Geometry check sheet. Reference: the model listing, model coordinates, mm. A direction names the side the tool comes from. Round coordinates to 2 decimals unless told otherwise and drop trailing zeros. Loops run counter-clockwise (first coordinate to the right, second up) from the corner with the lowest first, then second, coordinate; pieces in that order, holes last. Notation, with made-up numbers: M -31,84.25 L -17,84.25 A16 cw -17,107.25 Z; hole C 6.25,13.25 d8. An arc over 180 degrees is marked long. Answer in a Markdown table with one row per item. Add a question column.
```python
from build123d import *

# Parameters (mm, degrees)
SKETCH_1_R                = 31.85
EXTRUDE_1_DEPTH           = 18
SKETCH_2_R                = 25
SKETCH_2_R_2              = 9
CUT_EXTRUDE_1_DEPTH       = 6.2
CUT_EXTRUDE_START         = -6.2
SKETCH_3_R                = 25
SKETCH_3_R_2              = 9
CUT_EXTRUDE_5_DEPTH       = 6.2
EXTRUDE_START             = 9
SKETCH_4_R                = 9
EXTRUDE_2_DEPTH           = 9
SKETCH_5_R                = 3
CUT_EXTRUDE_6_DEPTH       = 53.515188279
SKETCH_6_R                = 6
CUT_EXTRUDE_7_DEPTH       = 48.538247759
CUT_EXTRUDE_10_REACH      = 60.414
CUT_EXTRUDE_10_END_RADIUS = 3
SKETCH_10_R               = 2
CUT_EXTRUDE_11_REACH      = 60.414
CUT_EXTRUDE_11_END_RADIUS = 3
SKETCH_7_R                = 2


with BuildPart() as part:
    # 草图1 → 凸台-拉伸1 (new body)
    with BuildSketch(Plane.XY):
        Circle(SKETCH_1_R)
    extrude(amount=EXTRUDE_1_DEPTH)

    # 草图2 → 切除-拉伸1 (cut)
    with BuildSketch(Plane.XY.offset(18)):
        Circle(SKETCH_2_R)
        Circle(SKETCH_2_R_2, mode=Mode.SUBTRACT)
    extrude(amount=-CUT_EXTRUDE_1_DEPTH, mode=Mode.SUBTRACT)

    # 草图3 → 切除-拉伸5 (cut)
    with BuildSketch(Plane(origin=(0, 0, 0), x_dir=(-1, 0, 0), z_dir=(0, 0, -1)).offset(CUT_EXTRUDE_START)):
        with Locations(Location((0, 0, 0), (0, 0, 180))):
            Circle(SKETCH_3_R)
        with Locations(Location((0, 0, 0), (0, 0, 180))):
            Circle(SKETCH_3_R_2, mode=Mode.SUBTRACT)
    extrude(amount=CUT_EXTRUDE_5_DEPTH, mode=Mode.SUBTRACT)

    # 草图4 → 凸台-拉伸2 (add)
    with BuildSketch(Plane.XY.offset(18).offset(EXTRUDE_START)):
        Circle(SKETCH_4_R)
    extrude(amount=-EXTRUDE_2_DEPTH)

    # 草图5 → 切除-拉伸6 (cut, through all)
    with BuildSketch(Plane.XY.offset(27)):
        Circle(SKETCH_5_R)
    extrude(amount=-CUT_EXTRUDE_6_DEPTH, mode=Mode.SUBTRACT)

    # 草图6 → 切除-拉伸7 (cut, through all)
    with BuildSketch(Plane.XY.offset(11.8)):
        with Locations((-17, 0)):
            Circle(SKETCH_6_R)
        with Locations((-8.5, 14.722431864)):
            Circle(SKETCH_6_R)
        with Locations((8.5, 14.722431864)):
            Circle(SKETCH_6_R)
        with Locations((17, 0)):
            Circle(SKETCH_6_R)
        with Locations((8.5, -14.722431864)):
            Circle(SKETCH_6_R)
        with Locations((-8.5, -14.722431864)):
            Circle(SKETCH_6_R)
    extrude(amount=-CUT_EXTRUDE_7_DEPTH, mode=Mode.SUBTRACT)

    # 切除-拉伸10: up to this cylinder (the profile starts outside it)
    cut_extrude_10_end = Plane(origin=(0, 0, 19.4), z_dir=(0, 0, 1)) * Cylinder(CUT_EXTRUDE_10_END_RADIUS, 127.828, mode=Mode.PRIVATE)
    # 草图10 → 切除-拉伸10 (cut, up to the surface)
    with BuildSketch(Plane(origin=(0, 9, 0), x_dir=(1, 0, 0), z_dir=(0, 1, 0)), mode=Mode.PRIVATE) as cut_extrude_10_sk1:
        with Locations(Location((0, -19.4, 0), (0, 0, 270))):
            Circle(SKETCH_10_R)
    cut_extrude_10_tool1 = extrude(cut_extrude_10_sk1.sketch, amount=-CUT_EXTRUDE_10_REACH, mode=Mode.PRIVATE) - cut_extrude_10_end
    add(cut_extrude_10_tool1.solids().sort_by_distance((0, 9, 19.4))[0], mode=Mode.SUBTRACT)

    # 切除-拉伸11: up to this cylinder (the profile starts outside it)
    cut_extrude_11_end = Plane(origin=(0, 0, 19.4), z_dir=(0, 0, 1)) * Cylinder(CUT_EXTRUDE_11_END_RADIUS, 127.828, mode=Mode.PRIVATE)
    # 草图7 → 切除-拉伸11 (cut, up to the surface)
    with BuildSketch(Plane(origin=(9, 0, 0), x_dir=(0, 0, -1), z_dir=(1, 0, 0)), mode=Mode.PRIVATE) as cut_extrude_11_sk1:
        with Locations((-19.4, 0)):
            Circle(SKETCH_7_R)
    cut_extrude_11_tool1 = extrude(cut_extrude_11_sk1.sketch, amount=-CUT_EXTRUDE_11_REACH, mode=Mode.PRIVATE) - cut_extrude_11_end
    add(cut_extrude_11_tool1.solids().sort_by_distance((9, 0, 19.4))[0], mode=Mode.SUBTRACT)


solid = part.part
```
1) Cross-section at A-A, the plane y = -15.5. Record the boundary of the cut face in (x, z).
2) Cross-section at D-D, the plane x = -20. Record the boundary of the cut face in (y, z), plus the area to 3 significant figures.
3) Cross-section at C-C, the plane y = 4.5. Count the separate pieces of the cut face and the enclosed holes in it, plus the area to 3 significant figures.
4) Go/stop test with flat-tipped pins: pin 1 (8 mm diameter, centred on x = -1.5, z = 4, fed in from -Y); pin 2 (2 mm diameter, centred on x = -15, z = 7.5, fed in from -Y); pin 3 (1 mm diameter, centred on y = -5, z = 20, fed in from +X). Record where each tip stops, or that it passes through.
5) Draft check along Y on faces 4 (the cylindrical face through (7.199, 8.865, 9.039)), 5 (the cylindrical face through (30.38, 9.57, 8.87)), 6 (the flat face through (0, -4, 0)). Enter one of: +Y half, -Y half, draft (parallel to the pull), parting line (faces both ways), or undercut.
6) Set-up check for faces 1 (the cylindrical face through (-0.766, 5.666, 21.247)), 2 (the cylindrical face through (23.846, 7.509, 14.943)), 3 (the flat face through (10.8, -0.4, 6.2)): record each of +Z, -Z, +X, -X, +Y, -Y from which the full face is reachable in a straight line by a thin tool's end or side.
7) Thickness scan on L1, parallel to Y at x = 0, z = 2.25; L2, parallel to Y at x = 8.5, z = 7.65; L3, parallel to Y at x = -12, z = 9.25. Record the ranges inside material, lowest first. Write a range as [from, to].
8) Cross-section at B-B, the plane x = -13. Record the boundary of the cut face in (y, z).
Worked answers:
| question | item | result |
|---|---|---|
| 1 | outline | M -27.82,0 L -19.62,0 L -19.62,6.2 L -14.45,6.2 L -14.45,11.8 L -19.62,11.8 L -19.62,18 L -27.82,18 Z; M -2.55,6.2 L 2.55,6.2 L 2.55,11.8 L -2.55,11.8 Z; M 14.45,6.2 L 19.62,6.2 L 19.62,0 L 27.82,0 L 27.82,18 L 19.62,18 L 19.62,11.8 L 14.45,11.8 Z |
| 2 | outline | M -24.79,0 L -15,0 L -15,6.2 L -5.2,6.2 L -5.2,11.8 L -15,11.8 L -15,18 L -24.79,18 Z; M 5.2,6.2 L 15,6.2 L 15,0 L 24.79,0 L 24.79,18 L 15,18 L 15,11.8 L 5.2,11.8 Z |
| 2 | area | 462 mm2 |
| 3 | separate pieces | 3 |
| 3 | enclosed holes | 1 |
| 3 | area | 757 mm2 |
| 4 | pin 1 | stops at y = -31.85 |
| 4 | pin 2 | stops at y = -28.61 |
| 4 | pin 3 | stops at x = 7.79 |
| 5 | face 4 | undercut |
| 5 | face 5 | parting line |
| 5 | face 6 | draft |
| 6 | face 1 | none |
| 6 | face 2 | +Z |
| 6 | face 3 | -Z |
| 7 | L1 | y = [-31.85, -25], [-9, -3], [3, 9], [25, 31.85] |
| 7 | L2 | y = [-30.69, -20.72], [-8.72, 8.72], [20.72, 30.69] |
| 7 | L3 | y = [-29.5, -19.6], [-9.85, -3.32], [3.32, 9.85], [19.6, 29.5] |
| 8 | outline | M -29.08,0 L -21.35,0 L -21.35,6.2 L -18.69,6.2 L -18.69,11.8 L -21.35,11.8 L -21.35,18 L -29.08,18 Z; M -10.75,6.2 L -4.47,6.2 L -4.47,11.8 L -10.75,11.8 Z; M 4.47,6.2 L 10.75,6.2 L 10.75,11.8 L 4.47,11.8 Z; M 18.69,6.2 L 21.35,6.2 L 21.35,0 L 29.08,0 L 29.08,18 L 21.35,18 L 21.35,11.8 L 18.69,11.8 Z |
